from build123d import *

# Parameters (mm, degrees)
SKETCH1_W           = 120
SKETCH1_H           = 25
SKETCH1_R           = 4
BOSS_EXTRUDE1_DEPTH = 10
SKETCH2_W           = 120
SKETCH2_H           = 10
BOSS_EXTRUDE2_DEPTH = 50


with BuildPart() as part:
    # Sketch1 → Boss-Extrude1 (new body)
    with BuildSketch(Plane.XY):
        Rectangle(SKETCH1_W, SKETCH1_H)
        with Locations((50, 0)):
            Circle(SKETCH1_R, mode=Mode.SUBTRACT)
        with BuildLine():
            Line((-47.89, 4), (20, 4))
            ThreePointArc((20, 4), (24, 0), (20, -4))
            Line((20, -4), (-47.89, -4))
            ThreePointArc((-47.89, -4), (-51.89, 0), (-47.89, 4))
        make_face(mode=Mode.SUBTRACT)
    extrude(amount=BOSS_EXTRUDE1_DEPTH)

    # Sketch2 → Boss-Extrude2 (add)
    with BuildSketch(Plane(origin=(0, 0, 0), x_dir=(-1, 0, 0), z_dir=(0, 0, -1))):
        with Locations((0, -17.5)):
            Rectangle(SKETCH2_W, SKETCH2_H)
    extrude(amount=-BOSS_EXTRUDE2_DEPTH)


solid = part.part
Design review of the part built by this model. Coordinates are the model's own, in mm. A direction names the side the tool comes from. Coordinates: 2 decimals unless noted, no trailing zeros. Loops run counter-clockwise (first coordinate to the right, second up) from the corner with the lowest first, then second, coordinate; pieces in that order, holes last.
Item 1: Draft analysis for pull direction Y (two halves, no side actions). For faces 1 (the flat face through (1, -5, 0)), 2 (the flat face through (-1, 12.5, 5)), 3 (the flat face through (-14, 4, 5)), state which applies: pulls with the +Y half, pulls with the -Y half, needs draft (parallel to the pull), parting line crosses it, or undercut.
Completed:
face 1: needs draft
face 2: pulls with the +Y half
face 3: undercut
Item 2: For faces 4 (the cylindrical face through (-51.89, -0.09, 4.93)), 5 (the flat face through (60, -13, 19)), 6 (the flat face through (1, -12.5, 30)), list the 3-axis set-ups (+Z, -Z, +X, -X, +Y, -Y) from which the entire face can be reached by the end or side of a thin tool; tool diameter is ignored.
Completed:
face 4: +Z, -Z
face 5: +Z, -Z, +X, +Y, -Y
face 6: +Z, +X, -X, +Y
Item 3: Add section C-C (y = 0). Write out the cut boundary in (x, z).
Completed:
outline: (-60, 0) - (-51.89, 0) - (-51.89, 10) - (-60, 10) - close; (24, 0) - (46, 0) - (46, 10) - (24, 10) - close; (54, 0) - (60, 0) - (60, 10) - (54, 10) - close
Item 4: Clearance check with flat-ended pins moving along their axes: pin 1 (5 mm diameter, centred on x = -11, z = 18.5, fed in from +Y); pin 2 (6 mm diameter, centred on x = 2.5, y = 3.5, fed in from +Z). State where each tip first meets the part, or that it passes through.
Completed:
pin 1: stops at y = -12.5
pin 2: stops at z = 10
Item 5: Add section A-A (z = 4). Write out the cut boundary in (x, y).
Completed:
outline: (-60, -22.5) - (60, -22.5) - (60, 12.5) - (-60, 12.5) - close; hole (-47.89, -4) - (20, -4) arc R4 ccw to (20, 4) - (-47.89, 4) arc R4 ccw to start; hole circle Ø8 at (50, 0)
Item 6: Wall thickness on L1, parallel to Y at x = 50, z = 7; L2, parallel to Z at x = 54, y = 7.5; L3, parallel to Y at x = 10, z = 37: over which ranges is each line inside the solid? List them lowest first.
Completed:
L1: y = -22.5 to -4, 4 to 12.5
L2: z = 0 to 10
L3: y = -22.5 to -12.5
Item 7: Add section B-B (x = -12.5). Write out the cut boundary in (y, z).
Completed:
outline: (-22.5, 0) - (-4, 0) - (-4, 10) - (-12.5, 10) - (-12.5, 50) - (-22.5, 50) - close; (4, 0) - (12.5, 0) - (12.5, 10) - (4, 10) - close
Item 8: Add section D-D (x = 22). Write out the cut boundary in (y, z).
Completed:
outline: (-22.5, 0) - (-3.46, 0) - (-3.46, 10) - (-12.5, 10) - (-12.5, 50) - (-22.5, 50) - close; (3.46, 0) - (12.5, 0) - (12.5, 10) - (3.46, 10) - close
